Geometry: final body of the model. Coordinates: model frame, mm. A direction names the side the tool comes from. Round coordinates to 2 decimals unless told otherwise and drop trailing zeros. Loops run counter-clockwise (first coordinate to the right, second up) from the corner with the lowest first, then second, coordinate; pieces in that order, holes last. Notation, with made-up numbers: (76, 73.25) - (130, 73.25) arc R30 cw to (130, 98.25) - close; hole circle Ø4 at (-19.75, 88.25). An arc over 180 degrees is marked (long way). Answer as a JSON object with one key per item and string values. Group by question number.
Item 1: Section C-C (z = -88.5). Return the cut outline in (x, y) (3 decimals).
Item 2: Line query: line 1 (X direction, y = 0.5, z = -100.5); line 2 (X direction, y = 1.05, z = -116); line 3 (X direction, y = 1.8, z = -141.5). Output: solid intervals per line, ascending.
Item 3: Reachability of faces 5 (the face through (-15.147, 1.565, -121.535)), 6 (the face through (-7, 0, -116)) from +Z, -Z, +X, -X, +Y, -Y: full face, straight path, thin tool, end or side. Return the list, or none.
Item 4: Section A-A (x = 0). Count the separate pieces of the cut face and the enclosed holes in it, plus the area to 3 significant figures.
Item 5: Draft query along X for faces 1 (the face through (10.662, 1.565, -143.042)), 2 (the face through (26.92, 1.57, -64.99)), 3 (the face through (-26.979, 1.565, -65.133)), 4 (the face through (-7, 3.175, -116)). Return one class per face: released by +X, released by -X, zero draft, split by the parting line, or undercut.
Item 6: Section B-B (z = -103). Return the cut outline in (x, y) (3 decimals).
```python
from build123d import *

# Parameters (mm, degrees)
SKETCH1_R           = 1.25
SKETCH1_R_2         = 1.5875
SKETCH1_R_3         = 6.35
SKETCH1_R_4         = 1.587499999
BOSS_EXTRUDE1_DEPTH = 3.175


with BuildPart() as part:
    # Sketch1 → Boss-Extrude1 (new body)
    with BuildSketch(Plane(origin=(0, 0, 0), x_dir=(1, 0, 0), z_dir=(0, 1, 0))):
        with BuildLine():
            Line((-19.061691445, 152.305177286), (-29.109279467, 70.814859111))
            ThreePointArc((-29.109279467, 70.814859111), (-29.106764186, 70.406916612), (-29.000369251, 70.01308476))
            Line((-29.000369251, 70.01308476), (-24.900498144, 60.115120329))
            ThreePointArc((-24.900498144, 60.115120329), (-24.059191565, 59.263489811), (-22.862282328, 59.241590515))
            ThreePointArc((-22.862282328, 59.241590515), (0, 63.5), (22.862282328, 59.241590515))
            ThreePointArc((22.862282328, 59.241590515), (24.059191565, 59.263489811), (24.900498144, 60.115120329))
            Line((24.900498144, 60.115120329), (29.000369251, 70.01308476))
            ThreePointArc((29.000369251, 70.01308476), (29.106764186, 70.406916612), (29.109279467, 70.814859111))
            Line((29.109279467, 70.814859111), (19.061691445, 152.305177286))
            ThreePointArc((19.061691445, 152.305177286), (19.052985039, 152.398309253), (19.049778848, 152.491792328))
            ThreePointArc((19.049778848, 152.491792328), (0, 171.45), (-19.049778848, 152.491792328))
            ThreePointArc((-19.049778848, 152.491792328), (-19.052985039, 152.398309253), (-19.061691445, 152.305177286))
        make_face()
        with Locations(Location((-10.606601718, 163.006601718, 0), (0, 0, 270))):
            Circle(SKETCH1_R, mode=Mode.SUBTRACT)
        with Locations(Location((0, 69.85, 0), (0, 0, 270))):
            Circle(SKETCH1_R_2, mode=Mode.SUBTRACT)
        with Locations(Location((18.0785103, 67.469918962, 0), (0, 0, 270))):
            Circle(SKETCH1_R_2, mode=Mode.SUBTRACT)
        with Locations(Location((10.606601718, 163.006601718, 0), (0, 0, 270))):
            Circle(SKETCH1_R, mode=Mode.SUBTRACT)
        with Locations(Location((10.606601718, 141.793398282, 0), (0, 0, 270))):
            Circle(SKETCH1_R, mode=Mode.SUBTRACT)
        with Locations(Location((0, 152.4, 0), (0, 0, 270))):
            Circle(SKETCH1_R_3, mode=Mode.SUBTRACT)
        with Locations(Location((-10.606601718, 141.793398282, 0), (0, 0, 270))):
            Circle(SKETCH1_R, mode=Mode.SUBTRACT)
        with Locations(Location((-18.078510302, 67.469918971, 0), (0, 0, 270))):
            Circle(SKETCH1_R_4, mode=Mode.SUBTRACT)
        with BuildLine():
            Line((-13.497810395, 120.266290898), (-4.865408959, 77.838541906))
            ThreePointArc((-4.865408959, 77.838541906), (-5.15124286, 76.569257194), (-6.289995152, 75.939949704))
            ThreePointArc((-6.289995152, 75.939949704), (-13.288948331, 75.032285399), (-20.173905346, 73.480974021))
            ThreePointArc((-20.173905346, 73.480974021), (-21.632306598, 73.810794489), (-22.169764015, 75.206092049))
            Line((-22.169764015, 75.206092049), (-16.629007128, 120.144045384))
            ThreePointArc((-16.629007128, 120.144045384), (-15.115368796, 121.53607252), (-13.497810395, 120.266290898))
        make_face(mode=Mode.SUBTRACT)
        with BuildLine():
            Line((-9.626782179, 133.089731304), (-1.555627758, 93.42047862))
            ThreePointArc((-1.555627758, 93.42047862), (0, 92.149488537), (1.555627758, 93.42047862))
            Line((1.555627758, 93.42047862), (9.626782179, 133.089731304))
            ThreePointArc((9.626782179, 133.089731304), (9.075338598, 134.635781943), (7.450296388, 134.867299588))
            ThreePointArc((7.450296388, 134.867299588), (0, 133.35), (-7.450296388, 134.867299588))
            ThreePointArc((-7.450296388, 134.867299588), (-9.075338598, 134.635781943), (-9.626782179, 133.089731304))
        make_face(mode=Mode.SUBTRACT)
        with BuildLine():
            Line((4.865408959, 77.838541906), (13.497810395, 120.266290898))
            ThreePointArc((13.497810395, 120.266290898), (15.115368796, 121.53607252), (16.629007128, 120.144045384))
            Line((16.629007128, 120.144045384), (22.169764015, 75.206092049))
            ThreePointArc((22.169764015, 75.206092049), (21.632306598, 73.810794489), (20.173905346, 73.480974021))
            ThreePointArc((20.173905346, 73.480974021), (13.288948331, 75.032285399), (6.289995152, 75.939949704))
            ThreePointArc((6.289995152, 75.939949704), (5.15124286, 76.569257194), (4.865408959, 77.838541906))
        make_face(mode=Mode.SUBTRACT)
    extrude(amount=BOSS_EXTRUDE1_DEPTH)


solid = part.part
```
Values:
{
 "1": {"outline": "(-26.929, 0) - (-20.531, 0) - (-20.531, 3.175) - (-26.929, 3.175) - close; (-7.035, 0) - (7.035, 0) - (7.035, 3.175) - (-7.035, 3.175) - close; (20.531, 0) - (26.929, 0) - (26.929, 3.175) - (20.531, 3.175) - close"},
 "2": {"line 1": "x = -25.45 to -19.05, -9.48 to -3, 3 to 9.48, 19.05 to 25.45", "line 2": "x = -23.54 to -17.14, -12.63 to -6.15, 6.15 to 12.63, 17.14 to 23.54", "line 3": "x = -20.39 to -11.82, -9.39 to 9.39, 11.82 to 20.39"},
 "3": {"face 5": "+Y, -Y", "face 6": "+Z, -Z, +X, -X, -Y"},
 "4": {"separate pieces": "4", "enclosed holes": "0", "area": "162 mm^2"},
 "5": {"face 1": "undercut", "face 2": "released by +X", "face 3": "released by -X", "face 4": "zero draft"},
 "6": {"outline": "(-25.141, 0) - (-18.743, 0) - (-18.743, 3.175) - (-25.141, 3.175) - close; (-9.985, 0) - (-3.505, 0) - (-3.505, 3.175) - (-9.985, 3.175) - close; (3.505, 0) - (9.985, 0) - (9.985, 3.175) - (3.505, 3.175) - close; (18.743, 0) - (25.141, 0) - (25.141, 3.175) - (18.743, 3.175) - close"}
}
